Geometry check sheet. Reference: the model listing, model coordinates, mm. A direction names the side the tool comes from. Coordinates: 2 decimals unless noted, no trailing zeros. Write each loop counter-clockwise with the first axis right and the second up, starting at its lowest first coordinate (ties: lowest second). Pieces come first, ordered by that corner, then holes. Notation, with made-up numbers: (34, 26) -> (75, 26) arc R19 ccw to (75, 33) -> close; hole circle Ø6 at (48, 2.5). An arc over 180 degrees is marked (long way). Answer in a Markdown table with one row per item. Add a question column.
Q1. Gauge pin test, flat ends, axial feed: P1, Ø4.5, axis at x = 138.5, y = 58.5, coming from the +Z side; P2, Ø5, axis at x = 166.22, y = 59.33, coming from the -Z side; P3, Ø6, axis at x = 161.5, y = 4.5, coming from the -Z side; P4, Ø15.5, axis at x = 158.5, z = 185, coming from the -Y side. Record the tip position at first contact, or that the pin passes through.
Q2. Tool access check on faces 4 (the face through (142.835, 57.384, 198.986)), 5 (the face through (146, 70, 169)), 6 (the face through (159, 71, 200)), 7 (the face through (166, 59, 195)). Record the directions out of +Z, -Z, +X, -X, +Y, -Y that give a thin tool (end or side, any length) a straight path to the whole face; none if there is none.
Q3. Section check B-B, the plane z = 191.5. Record the boundary of the cut face in (x, y), and give its area (3 significant figures).
Q4. Section check C-C, the plane y = 15.5. Record the boundary of the cut face in (x, z), and give its area (3 significant figures).
Q5. Section check A-A, the plane x = 159.5. Record the boundary of the cut face in (y, z), and give its area (3 significant figures).
Q6. Thickness scan on line 1 (X direction, y = 97, z = 170); line 2 (Z direction, x = 135, y = 71); line 3 (Z direction, x = 158, y = 91). Record the ranges inside material, lowest first.
Q7. Release check for a two-part mould opening along Y. For faces 1 (the face through (138, 99, 195)), 2 (the face through (138, 99, 169)), 3 (the face through (133.1, 50.96, 184.69)) record: pulls with the +Y half, pulls with the -Y half, needs draft (parallel to the pull), parting line crosses it, or undercut.
```python
from build123d import *

# Parameters (mm, degrees)
SKETCH1_W           = 40
SKETCH1_H           = 58.200000762
BOSS_EXTRUDE1_DEPTH = 27
SKETCH2_R           = 15.499999921
BOSS_EXTRUDE2_DEPTH = 57
SKETCH3_R           = 9.900000829
BOSS_EXTRUDE3_DEPTH = 4.5
SKETCH4_R           = 3.999999654
BOSS_EXTRUDE4_DEPTH = 15
CUT_EXTRUDE1_DEPTH  = 13
BOSS_EXTRUDE5_DEPTH = 2
BOSS_EXTRUDE6_DEPTH = 2
BOSS_EXTRUDE7_DEPTH = 2
SKETCH9_W           = 4.500000339
SKETCH9_H           = 2
SKETCH10_W          = 4.500000226
SKETCH10_H          = 2
SKETCH11_W          = 4.499999816
SKETCH11_H          = 2
SKETCH12_W          = 4.500000657
SKETCH12_H          = 2
SKETCH13_W          = 4.49999985
SKETCH13_H          = 2
SKETCH14_W          = 9.899999781
SKETCH14_H          = 4.5
SKETCH15_W          = 4.500000004
SKETCH15_H          = 2
SKETCH16_W          = 4.49999905
SKETCH16_H          = 2
SKETCH17_W          = 4.499999637
SKETCH17_H          = 2
SKETCH18_W          = 4.500001132
SKETCH18_H          = 2
SKETCH19_W          = 4.499999489
SKETCH19_H          = 2
FILLET1_R           = 2.913033302
SKETCH20_R          = 2
CUT_EXTRUDE2_DEPTH  = 5


with BuildPart() as part:
    # Sketch1 → Boss-Extrude1 (new body)
    with BuildSketch(Plane(origin=(0, 0, 171), x_dir=(-1, 0, 0), z_dir=(0, 0, -1))):
        with Locations((-152.219146729, 79.232439518)):
            Rectangle(SKETCH1_W, SKETCH1_H)
    extrude(amount=-BOSS_EXTRUDE1_DEPTH)

    # Sketch2 → Boss-Extrude2 (add)
    with BuildSketch(Plane.XZ.offset(-50.132439137)):
        with Locations((152.219146662, 180.000000025)):
            Circle(SKETCH2_R)
    extrude(amount=BOSS_EXTRUDE2_DEPTH)

    # Sketch3 → Boss-Extrude3 (add)
    with BuildSketch(Plane.XY.offset(198)):
        with Locations((152.21914569, 88.232439899)):
            Circle(SKETCH3_R)
    extrude(amount=BOSS_EXTRUDE3_DEPTH)

    # Sketch4 → Boss-Extrude4 (add)
    with BuildSketch(Plane.XY.offset(202.5)):
        with Locations((152.219146674, 88.232439899)):
            Circle(SKETCH4_R)
    extrude(amount=BOSS_EXTRUDE4_DEPTH)

    # Sketch5 → Cut-Extrude1 (cut)
    with BuildSketch(Plane.XY.offset(217.5)):
        with BuildLine():
            Line((149.573395252, 91.232439899), (154.864898205, 91.232439899))
            ThreePointArc((154.864898205, 91.232439899), (152.219146729, 92.232440009), (149.573395252, 91.232439899))
        make_face()
    extrude(amount=-CUT_EXTRUDE1_DEPTH, mode=Mode.SUBTRACT)

    # Sketch6 → Boss-Extrude5 (add)
    with BuildSketch(Plane.XY.offset(198)):
        with BuildLine():
            Line((135.03716583, 62.314419458), (137.865592743, 65.142846371))
            ThreePointArc((137.865592743, 65.142846371), (144.229553368, 65.142846505), (144.22955377, 58.778885881))
            Line((144.22955377, 58.778885881), (141.401127095, 55.95045873))
            ThreePointArc((141.401127095, 55.95045873), (135.037165964, 55.950458327), (135.03716583, 62.314419458))
        make_face()
    extrude(amount=BOSS_EXTRUDE5_DEPTH)

    # Sketch7 → Boss-Extrude6 (add)
    with BuildSketch(Plane(origin=(0, 0, 171), x_dir=(-1, 0, 0), z_dir=(0, 0, -1))):
        with BuildLine():
            ThreePointArc((-142.483799553, 57.696214596), (-144.229553379, 65.142847459), (-136.782921252, 63.397090493))
            ThreePointArc((-136.782921252, 63.397090493), (-135.037167167, 55.950457372), (-142.483799553, 57.696214596))
        make_face()
    extrude(amount=BOSS_EXTRUDE6_DEPTH)

    # Sketch8 → Boss-Extrude7 (add)
    with BuildSketch(Plane.XZ.offset(6.867560863)):
        with BuildLine():
            Line((158.212552085, 179.71876642), (158.159881829, 179.158770706))
            ThreePointArc((158.159881829, 179.158770706), (146.245510806, 180.561848666), (158.212552085, 179.71876642))
        make_face()
    extrude(amount=BOSS_EXTRUDE7_DEPTH)

    # Sketch9 → Revolve1 (revolve)
    with BuildSketch(Plane.XZ.offset(-59.132439085)):
        with Locations((168.469147961, 170)):
            Rectangle(SKETCH9_W, SKETCH9_H)
    revolve(axis=Axis((166.219147791, 59.132439085, 171), (0, 0, -1)))

    # Sketch10 → Revolve2 (revolve)
    with BuildSketch(Plane.XZ.offset(-99.132437815)):
        with Locations((140.469147187, 170)):
            Rectangle(SKETCH10_W, SKETCH10_H)
    revolve(axis=Axis((138.219147074, 99.132437815, 171), (0, 0, -1)))

    # Sketch11 → Revolve3 (revolve)
    with BuildSketch(Plane.XZ.offset(-70.532439222)):
        with Locations((160.769146188, 170)):
            Rectangle(SKETCH11_W, SKETCH11_H)
    revolve(axis=Axis((158.51914628, 70.532439222, 171), (0, 0, -1)))

    # Sketch12 → Revolve4 (revolve)
    with BuildSketch(Plane.XZ.offset(-99.132437815)):
        with Locations((168.46914727, 170)):
            Rectangle(SKETCH12_W, SKETCH12_H)
    revolve(axis=Axis((166.219146941, 99.132437815, 171), (0, 0, -1)))

    # Sketch13 → Revolve5 (revolve)
    with BuildSketch(Plane.XZ.offset(-70.532439222)):
        with Locations((148.16914686, 170)):
            Rectangle(SKETCH13_W, SKETCH13_H)
    revolve(axis=Axis((145.919146935, 70.532439222, 171), (0, 0, -1)))

    # Sketch14 → Revolve6 (revolve)
    with BuildSketch(Plane.XZ.offset(-88.232439085)):
        with Locations((157.169146737, 168.75)):
            Rectangle(SKETCH14_W, SKETCH14_H)
    revolve(axis=Axis((152.219146846, 88.232439085, 171), (0, 0, -1)))

    # Sketch15 → Revolve7 (revolve)
    with BuildSketch(Plane(origin=(0, 59.332439899, 0), x_dir=(1, 0, 0), z_dir=(0, 1, 0))):
        with Locations((168.469147213, -199)):
            Rectangle(SKETCH15_W, SKETCH15_H)
    revolve(axis=Axis((166.219147211, 59.332439899, 198), (0, 0, 1)))

    # Sketch16 → Revolve8 (revolve)
    with BuildSketch(Plane(origin=(0, 99.332439899, 0), x_dir=(1, 0, 0), z_dir=(0, 1, 0))):
        with Locations((168.469146681, -199)):
            Rectangle(SKETCH16_W, SKETCH16_H)
    revolve(axis=Axis((166.219147156, 99.332439899, 198), (0, 0, 1)))

    # Sketch17 → Revolve9 (revolve)
    with BuildSketch(Plane(origin=(0, 70.532438002, 0), x_dir=(1, 0, 0), z_dir=(0, 1, 0))):
        with Locations((160.769147041, -199)):
            Rectangle(SKETCH17_W, SKETCH17_H)
    revolve(axis=Axis((158.519147223, 70.532438002, 198), (0, 0, 1)))

    # Sketch18 → Revolve10 (revolve)
    with BuildSketch(Plane(origin=(0, 99.332439899, 0), x_dir=(1, 0, 0), z_dir=(0, 1, 0))):
        with Locations((140.469146163, -199)):
            Rectangle(SKETCH18_W, SKETCH18_H)
    revolve(axis=Axis((138.219145597, 99.332439899, 198), (0, 0, 1)))

    # Sketch19 → Revolve11 (revolve)
    with BuildSketch(Plane(origin=(0, 70.532438002, 0), x_dir=(1, 0, 0), z_dir=(0, 1, 0))):
        with Locations((148.169147032, -199)):
            Rectangle(SKETCH19_W, SKETCH19_H)
    revolve(axis=Axis((145.919147287, 70.532438002, 198), (0, 0, 1)))

    # Fillet1
    fillet1_edges = [part.edges().sort_by_distance(p)[0] for p in [
        (132.219146729, 108.332439899, 184.5),
        (132.219146729, 50.132439137, 184.5),
        (172.219146729, 50.132439137, 184.5),
        (172.219146729, 108.332439899, 184.5),
    ]]
    fillet(fillet1_edges, radius=FILLET1_R)

    # Sketch20 → Cut-Extrude2 (cut)
    with BuildSketch(Plane.XY.offset(200)):
        with Locations((138.219145597, 99.332439899)):
            Circle(SKETCH20_R)
        with Locations((166.219147211, 99.332439899)):
            Circle(SKETCH20_R)
        with Locations((138.219145597, 59.332439899)):
            Circle(SKETCH20_R)
        with Locations((166.219147211, 59.332439899)):
            Circle(SKETCH20_R)
    extrude(amount=-CUT_EXTRUDE2_DEPTH, mode=Mode.SUBTRACT)


solid = part.part
```
Calculated:
| question | item | result |
|---|---|---|
| 1 | P1 | stops at z = 200 |
| 1 | P2 | stops at z = 169 |
| 1 | P3 | stops at z = 165.83 |
| 1 | P4 | stops at y = -8.87 |
| 2 | face 4 | +Z, -Y |
| 2 | face 5 | -Z, +X, -X |
| 2 | face 6 | +Z, +X, -X, -Y |
| 2 | face 7 | +Z |
| 3 | outline | (132.22, 53.05) arc R2.91 ccw to (135.13, 50.13) -> (141.83, 50.13) -> (141.83, -6.87) -> (162.61, -6.87) -> (162.61, 50.13) -> (169.31, 50.13) arc R2.91 ccw to (172.22, 53.05) -> (172.22, 105.42) arc R2.91 ccw to (169.31, 108.33) -> (135.13, 108.33) arc R2.91 ccw to (132.22, 105.42) -> close |
| 3 | area | 3,510 mm² |
| 4 | outline | circle Ø31 at (152.22, 180) |
| 4 | area | 755 mm² |
| 5 | outline | (-6.87, 166.32) -> (50.13, 166.32) -> (50.13, 171) -> (66.14, 171) -> (66.14, 169) -> (74.92, 169) -> (74.92, 171) -> (81.52, 171) -> (81.52, 166.5) -> (94.94, 166.5) -> (94.94, 171) -> (108.33, 171) -> (108.33, 198) -> (94.94, 198) -> (94.94, 202.5) -> (81.52, 202.5) -> (81.52, 198) -> (74.92, 198) -> (74.92, 200) -> (66.14, 200) -> (66.14, 198) -> (50.13, 198) -> (50.13, 193.68) -> (-6.87, 193.68) -> close |
| 5 | area | 3,290 mm² |
| 6 | line 1 | x = 134.26 to 142.18, 147.62 to 156.82, 162.26 to 170.18 |
| 6 | line 2 | z = 171 to 198 |
| 6 | line 3 | z = 166.5 to 202.5 |
| 7 | face 1 | undercut |
| 7 | face 2 | needs draft |
| 7 | face 3 | pulls with the -Y half |
